from build123d import *

# Parameters (mm, degrees)
SKETCH1_W               = 101.6
SKETCH1_H               = 101.6
SKETCH1_R               = 4.318
BOSS_EXTRUDE1_DEPTH     = 12.7
SKETCH2_R               = 38.1
BOSS_EXTRUDE2_DEPTH     = 3.81
SKETCH4_R               = 7.9375
BOSS_EXTRUDE4_DEPTH     = 39.37
CUT_EXTRUDE1_DEPTH      = 1
CUT_EXTRUDE1_DEPTH_BACK = 39.37
SKETCH6_R               = 50.8
BOSS_EXTRUDE5_DEPTH     = 160.782
SKETCH7_R               = 38.1
BOSS_EXTRUDE6_DEPTH     = 3.81
SKETCH8_R               = 6.35
BOSS_EXTRUDE7_DEPTH     = 17.78


with BuildPart() as part:
    # Sketch1 → Boss-Extrude1 (new body)
    with BuildSketch(Plane.XY):
        Rectangle(SKETCH1_W, SKETCH1_H)
        with Locations((-43.18, -43.18)):
            Circle(SKETCH1_R, mode=Mode.SUBTRACT)
        with Locations((43.18, -43.18)):
            Circle(SKETCH1_R, mode=Mode.SUBTRACT)
        with Locations((43.18, 43.18)):
            Circle(SKETCH1_R, mode=Mode.SUBTRACT)
        with Locations((-43.18, 43.18)):
            Circle(SKETCH1_R, mode=Mode.SUBTRACT)
    extrude(amount=BOSS_EXTRUDE1_DEPTH)

    # Sketch2 → Boss-Extrude2 (add)
    with BuildSketch(Plane.XY.offset(12.7)):
        Circle(SKETCH2_R)
    extrude(amount=BOSS_EXTRUDE2_DEPTH)

    # Sketch4 → Boss-Extrude4 (add)
    with BuildSketch(Plane.XY.offset(16.51)):
        Circle(SKETCH4_R)
    extrude(amount=BOSS_EXTRUDE4_DEPTH)

    # Sketch5 → Cut-Extrude1 (cut, two sides)
    with BuildSketch(Plane.XY.offset(55.88)) as cut_extrude1_sk:
        with BuildLine():
            Line((-2.387594518, 5.063803231), (5.482e-06, 5.063803231))
            Line((5.482e-06, 5.063803231), (2.387605482, 5.063803231))
            Line((2.387605482, 5.063803231), (2.387605482, 7.569890773))
            ThreePointArc((2.387605482, 7.569890773), (5.748e-06, 7.9375), (-2.387594518, 7.569894231))
            Line((-2.387594518, 7.569894231), (-2.387594518, 5.063803231))
        make_face()
    extrude(amount=CUT_EXTRUDE1_DEPTH, mode=Mode.SUBTRACT)
    extrude(cut_extrude1_sk.sketch, amount=-CUT_EXTRUDE1_DEPTH_BACK, mode=Mode.SUBTRACT)

    # Sketch6 → Boss-Extrude5 (add)
    with BuildSketch(Plane(origin=(0, 0, 0), x_dir=(-1, 0, 0), z_dir=(0, 0, -1))):
        Circle(SKETCH6_R)
    extrude(amount=BOSS_EXTRUDE5_DEPTH)

    # Sketch7 → Boss-Extrude6 (add)
    with BuildSketch(Plane(origin=(0, 0, -160.782), x_dir=(-1, 0, 0), z_dir=(0, 0, -1))):
        Circle(SKETCH7_R)
    extrude(amount=BOSS_EXTRUDE6_DEPTH)

    # Sketch8 → Boss-Extrude7 (add)
    with BuildSketch(Plane(origin=(0, 0, -164.592), x_dir=(-1, 0, 0), z_dir=(0, 0, -1))):
        Circle(SKETCH8_R)
    extrude(amount=BOSS_EXTRUDE7_DEPTH)


solid = part.part
The listing builds one solid part. Answer for the finished solid, in the listing's coordinates (mm). A direction names the side the tool comes from. Coordinates: 2 decimals unless noted, no trailing zeros. Loops run counter-clockwise (first coordinate to the right, second up) from the corner with the lowest first, then second, coordinate; pieces in that order, holes last. Notation, with made-up numbers: (2.5, 9) -> (51.5, 9) arc R29 cw to (51.5, 43) -> close; hole circle Ø1 at (34, 48). An arc over 180 degrees is marked (long way). Answer in a Markdown table with one row per item. Add a question column.
1. The part is cut by section D-D, the plane z = -117.5. Write down the section's boundary in (x, y).
2. The part is cut by section A-A, the plane x = -43.18. Write down the section's boundary in (y, z).
3. For faces 1 (the flat face through (38, 39, 0)), 2 (the flat face through (22, 35, 12.7)), 3 (the cylindrical face through (30.235, -23.183, -162.66)), 4 (the flat face through (38, -40, 0)), determine the directions among +Z, -Z, +X, -X, +Y, -Y from which every point of the face is accessible in a straight line to the end or side of a thin tool.
4. Flat-ended cylindrical pins translate along their axes: P1, Ø5, axis at x = 17, y = -16, coming from the -Z side; P2, Ø1, axis at y = -16, z = -105, coming from the -X side; P3, Ø11, axis at x = 43.18, y = -43.18, coming from the +Z side. Find the tip coordinate at first contact, or state that the pin passes through.
5. The part is cut by section C-C, the plane y = 29. Write down the section's boundary in (x, z).
6. Determine the mould class of faces 5 (the flat face through (-39, 39, 0)), 6 (the flat face through (0, 5.064, 36)), 7 (the cylindrical face through (11.012, -49.592, -79.266)) for opening direction X: +X half, -X half, draft (parallel to the pull), parting line (faces both ways), or undercut.
7. Consider line 1 (Y direction, x = -43, z = 6); line 2 (Z direction, x = -2.5, y = 17). Determine where each line is inside the solid, lowest interval first. Write a range as [from, to].
Answer below:
| question | item | result |
|---|---|---|
| 1 | outline | circle Ø101.6 at (0, 0) |
| 2 | outline | (-50.8, 0) -> (-47.5, 0) -> (-47.5, 12.7) -> (-50.8, 12.7) -> close; (-38.86, 0) -> (-26.76, 0) -> (-26.76, -160.78) -> (26.76, -160.78) -> (26.76, 0) -> (38.86, 0) -> (38.86, 12.7) -> (-38.86, 12.7) -> close; (47.5, 0) -> (50.8, 0) -> (50.8, 12.7) -> (47.5, 12.7) -> close |
| 3 | face 1 | -Z, +X, +Y |
| 3 | face 2 | +Z |
| 3 | face 3 | -Z |
| 3 | face 4 | -Z, +X, -Y |
| 4 | P1 | z = -164.59 |
| 4 | P2 | x = -48.38 |
| 4 | P3 | z = 12.7 |
| 5 | outline | (-50.8, 0) -> (-41.71, 0) -> (-41.71, -160.78) -> (-24.71, -160.78) -> (-24.71, -164.59) -> (24.71, -164.59) -> (24.71, -160.78) -> (41.71, -160.78) -> (41.71, 0) -> (50.8, 0) -> (50.8, 12.7) -> (24.71, 12.7) -> (24.71, 16.51) -> (-24.71, 16.51) -> (-24.71, 12.7) -> (-50.8, 12.7) -> close |
| 6 | face 5 | draft |
| 6 | face 6 | undercut |
| 6 | face 7 | parting line |
| 7 | line 1 | [-50.8, -47.49], [-38.87, 38.87], [47.49, 50.8] |
| 7 | line 2 | [-164.59, 16.51] |
